Input: part model. Units: mm. Frame: model coordinates. A direction names the side the tool comes from. Coordinates: 2 decimals unless noted, no trailing zeros. Write each loop counter-clockwise with the first axis right and the second up, starting at its lowest first coordinate (ties: lowest second). Pieces come first, ordered by that corner, then holes.
1) Set-up query: faces 1 (the flat face through (0, -2.5, 1)), 2 (the flat face through (22, 18, 7)), 3 (the flat face through (0, 24, 10)), 4 (the flat face through (-23.9, -16.6, 3)), 5 (the flat face through (23, -15.5, 1)). Return all of +Z, -Z, +X, -X, +Y, -Y with unobstructed straight access to the full face (end or side cutting, diameter ignored); none if empty.
2) Section query D-D (x = -16). Output: boundary loops of the cut face in (y, z), then the cut area to 3 significant figures.
3) Draft query along Y for faces 6 (the flat face through (-10, 0, 2)), 7 (the flat face through (16, -5, 8)), 8 (the flat face through (20, 17, 5)). Return one class per face: pulls with the +Y half, pulls with the -Y half, needs draft (parallel to the pull), parting line crosses it, or undercut.
4) Section query B-B (x = -2). Output: boundary loops of the cut face in (y, z), then the cut area to 3 significant figures.
5) Pin query (flat end, axial travel): pin 1 Ø0.8 at (x, y) = (22.5, 17.5) entering from -Z; pin 2 Ø2.5 at (x, z) = (-16, 9) entering from -Y; pin 3 Ø10 at (x, y) = (-17.5, 11) entering from +Z. Return the tip coordinate at first contact, or that it passes through.
6) Section query C-C (y = -17.5). Output: boundary loops of the cut face in (x, z).
7) Line query: L1, parallel to X at y = 2, z = 7.5; L2, parallel to X at y = 18, z = 16; L3, parallel to X at y = 20, z = 4.5. Output: solid intervals per line, ascending.
from build123d import *

# Parameters (mm, degrees)
SKICA1_W                  = 50
SKICA1_H                  = 50
P_IDAT_VYSUNUT_M2_DEPTH   = 3
SKICA4_W                  = 20
SKICA4_H                  = 5
ODEBRAT_VYSUNUT_M1_DEPTH  = 2
SKICA5_W                  = 50
SKICA5_H                  = 5
ODEBRAT_VYSUNUT_M3_DEPTH  = 1
SKICA10_W                 = 5
SKICA10_H                 = 10
P_IDAT_VYSUNUT_M6_DEPTH   = 10
ODEBRAT_VYSUNUT_M6_DEPTH  = 10
P_IDAT_VYSUNUT_M9_DEPTH   = 15
SKICA17_R                 = 2
ODEBRAT_VYSUNUT_M8_DEPTH  = 4
SKICA18_W                 = 5
SKICA18_H                 = 5
P_IDAT_VYSUNUT_M10_DEPTH  = 7
SKICA19_W                 = 4
SKICA19_H                 = 4
ODEBRAT_VYSUNUT_M10_DEPTH = 3
ZKOSEN_2_SIZE             = 4
SKICA20_R                 = 1.25
ODEBRAT_VYSUNUT_M11_DEPTH = 3


with BuildPart() as part:
    # Skica1 → Přidat vysunutím2 (new body)
    with BuildSketch(Plane.XY):
        Rectangle(SKICA1_W, SKICA1_H)
    extrude(amount=P_IDAT_VYSUNUT_M2_DEPTH)

    # Skica4 → Odebrat vysunutím1 (cut)
    with BuildSketch(Plane.XY.offset(3)):
        Rectangle(SKICA4_W, SKICA4_H)
    extrude(amount=-ODEBRAT_VYSUNUT_M1_DEPTH, mode=Mode.SUBTRACT)

    # Skica5 → Odebrat vysunutím3 (cut)
    with BuildSketch(Plane(origin=(0, 0, 0), x_dir=(-1, 0, 0), z_dir=(0, 0, -1))):
        Rectangle(SKICA5_W, SKICA5_H)
    extrude(amount=-ODEBRAT_VYSUNUT_M3_DEPTH, mode=Mode.SUBTRACT)

    # Skica10 → Přidat vysunutím6 (add)
    with BuildSketch(Plane.XY.offset(3)):
        with Locations((-16, 0)):
            Rectangle(SKICA10_W, SKICA10_H)
        with Locations((16, 0)):
            Rectangle(SKICA10_W, SKICA10_H)
    extrude(amount=P_IDAT_VYSUNUT_M6_DEPTH)

    # Skica12 → Odebrat vysunutím6 (cut)
    with BuildSketch(Plane(origin=(0, 5, 0), x_dir=(1, 0, 0), z_dir=(0, 1, 0))):
        Polygon((-13.5, -13), (-13.5, -11), (-15, -12), align=None)
        Polygon((13.5, -13), (13.5, -11), (15, -12), align=None)
    extrude(amount=-ODEBRAT_VYSUNUT_M6_DEPTH, mode=Mode.SUBTRACT)

    # Skica14 → Přidat vysunutím9 (add)
    with BuildSketch(Plane.XY.offset(3)):
        Polygon((25, 25), (-25, 25), (-25, -25), (-24, -25), (-24, 24), (24, 24), (24, -25), (25, -25), align=None)
    extrude(amount=P_IDAT_VYSUNUT_M9_DEPTH)

    # Skica17 → Odebrat vysunutím8 (cut)
    with BuildSketch(Plane(origin=(0, 0, 1), x_dir=(-1, 0, 0), z_dir=(0, 0, -1))):
        with Locations((-16, 0)):
            Circle(SKICA17_R)
        with Locations((16, 0)):
            Circle(SKICA17_R)
    extrude(amount=-ODEBRAT_VYSUNUT_M8_DEPTH, mode=Mode.SUBTRACT)

    # Skica18 → Přidat vysunutím10 (add)
    with BuildSketch(Plane(origin=(0, 0, 0), x_dir=(-1, 0, 0), z_dir=(0, 0, -1))):
        with Locations((-22.5, 17.5)):
            Rectangle(SKICA18_W, SKICA18_H)
        with Locations((22.5, 17.5)):
            Rectangle(SKICA18_W, SKICA18_H)
        with Locations((22.5, -17.5)):
            Rectangle(SKICA18_W, SKICA18_H)
        with Locations((-22.5, -17.5)):
            Rectangle(SKICA18_W, SKICA18_H)
    extrude(amount=-P_IDAT_VYSUNUT_M10_DEPTH)

    # Skica19 → Odebrat vysunutím10 (cut)
    with BuildSketch(Plane(origin=(0, 0, 0), x_dir=(-1, 0, 0), z_dir=(0, 0, -1))):
        with Locations((-23, -17.5)):
            Rectangle(SKICA19_W, SKICA19_H)
        with Locations((-23, 17.5)):
            Rectangle(SKICA19_W, SKICA19_H)
        with Locations((23, 17.5)):
            Rectangle(SKICA19_W, SKICA19_H)
        with Locations((23, -17.5)):
            Rectangle(SKICA19_W, SKICA19_H)
    extrude(amount=-ODEBRAT_VYSUNUT_M10_DEPTH, mode=Mode.SUBTRACT)

    # Zkosení2
    zkosen_2_edges = [part.edges().sort_by_distance(p)[0] for p in [
        (22, 15, 3),
        (22, 20, 3),
        (-22, 20, 3),
        (-22, 15, 3),
        (-22, -15, 3),
        (-22, -20, 3),
        (22, -20, 3),
        (22, -15, 3),
    ]]
    chamfer(zkosen_2_edges, length=ZKOSEN_2_SIZE - 0.0001)  # a hair under: the kernel refuses the full size

    # Skica20 → Odebrat vysunutím11 (cut)
    with BuildSketch(Plane(origin=(0, 0, 3), x_dir=(-1, 0, 0), z_dir=(0, 0, -1))):
        with Locations((22.75, 17.5)):
            Circle(SKICA20_R)
        with Locations(Location((22.75, -17.5, 0), (0, 0, 180))):
            Circle(SKICA20_R)
        with Locations((-22.75, -17.5)):
            Circle(SKICA20_R)
        with Locations(Location((-22.75, 17.5, 0), (0, 0, 180))):
            Circle(SKICA20_R)
    extrude(amount=-ODEBRAT_VYSUNUT_M11_DEPTH, mode=Mode.SUBTRACT)


solid = part.part
Answer:
1. face 1: -Z
1. face 2: +Z, -Y
1. face 3: +Z
1. face 4: -Z, -X
1. face 5: -Z, +X
2. outline: (-25, 0) - (-2.5, 0) - (-2.5, 1) - (-2, 1) - (-2, 5) - (2, 5) - (2, 1) - (2.5, 1) - (2.5, 0) - (25, 0) - (25, 18) - (24, 18) - (24, 3) - (5, 3) - (5, 13) - (-5, 13) - (-5, 3) - (-25, 3) - close
2. area: 244 mm2
3. face 6: undercut
3. face 7: pulls with the -Y half
3. face 8: needs draft
4. outline: (-25, 0) - (-2.5, 0) - (-2.5, 3) - (-25, 3) - close; (2.5, 0) - (25, 0) - (25, 18) - (24, 18) - (24, 3) - (2.5, 3) - close
4. area: 150 mm2
5. pin 1: stops at z = 6
5. pin 2: stops at y = -5
5. pin 3: stops at z = 7
6. outline: (-25, 3) - (-24, 3) - (-24, 6) - (-21.5, 6) - (-21.5, 3) - (-21, 3) - (-21, 0) - (21, 0) - (21, 3) - (21.5, 3) - (21.5, 6) - (24, 6) - (24, 3) - (25, 3) - (25, 18) - (24, 18) - (24, 7) - (20, 7) - (20, 3) - (-20, 3) - (-20, 7) - (-24, 7) - (-24, 18) - (-25, 18) - close
7. L1: x = -25 to -24, -18.5 to -13.5, 13.5 to 18.5, 24 to 25
7. L2: x = -25 to -24, 24 to 25
7. L3: x = -25 to -20, 20 to 25
